from build123d import *

# Parameters (mm, degrees)
F1_DEPTH = 7.25
F2_R     = 3
F3_DEPTH = 25


with BuildPart() as f1:
    # F0 (on Right) → F1 (new body, symmetric)
    with BuildSketch(Plane.YZ):
        with BuildLine():
            Line((14.5, 0), (14.1, 0))
            Line((14.1, 0), (14.1, -0.4))
            Line((14.1, -0.4), (14.1, -1.5))
            Line((14.1, -1.5), (0, -1.5))
            Line((0, -1.5), (0, -1.9))
            Line((0, -1.9), (14.5, -1.9))
            Line((14.5, -1.9), (14.5, -0.4))
            Line((14.5, -0.4), (39.5, -0.4))
            ThreePointArc((39.5, -0.4), (56.431793, 16.531793), (39.5, 33.463586))
            ThreePointArc((39.5, 33.463586), (25.182343, 18.203119), (39.5, 2.942652))
            Line((39.5, 2.942652), (39.5, 3.544018))
            ThreePointArc((39.5, 3.544018), (25.778463, 18.272009), (39.5, 33))
            ThreePointArc((39.5, 33), (56, 16.5), (39.5, 0))
            Line((39.5, 0), (14.5, 0))
        make_face()
    extrude(amount=F1_DEPTH, both=True)

    # F2 (on face) → F3 (cut)
    with BuildSketch(Plane.XY.offset(-1.5)):
        with BuildLine():
            ThreePointArc((6.233854, 1.274401), (3.159757, 0.427693), (0, 0))
            Line((0, 0), (7.25, 0))
            Line((7.25, 0), (7.25, 4.562755))
            Line((7.25, 4.562755), (6.233854, 1.274401))
        make_face()
        with BuildLine():
            ThreePointArc((0, 0), (-3.159757, 0.427693), (-6.233854, 1.274401))
            Line((-6.233854, 1.274401), (-7.25, 4.562755))
            Line((-7.25, 4.562755), (-7.25, 0))
            Line((-7.25, 0), (0, 0))
        make_face()
        with Locations((0, 6)):
            Circle(F2_R)
    extrude(amount=-F3_DEPTH, mode=Mode.SUBTRACT)


solid = f1.part
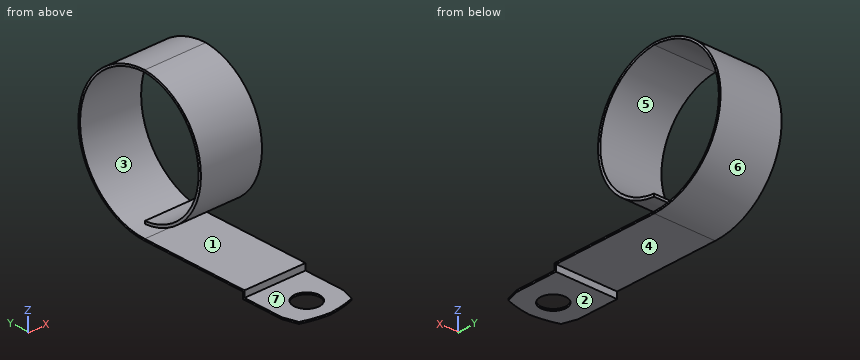
Check sheet for the modelled part. Datum: model origin and axes. Units: mm. Face numbers are marked on the shaded views. A direction names the side the tool comes from. Give positions to 0.01 mm unless a question says otherwise; leave off trailing zeros. Write each loop counter-clockwise with the first axis right and the second up, starting at its lowest first coordinate (ties: lowest second). Pieces come first, ordered by that corner, then holes. Notation, with made-up numbers: (49, 51.5) -> (106, 51.5) arc R18 ccw to (106, 62.5) -> close; hole circle Ø7 at (53.25, 38.5). An arc over 180 degrees is marked (long way). Use one line per item in the form item = value. Start each with the question number.
1. Mould release check, pull along Y, two halves, no side actions. Record for the marked faces 5, 6 and 7: pulls with the +Y half, pulls with the -Y half, needs draft (parallel to the pull), parting line crosses it, or undercut.
2. Access from +Z, -Z, +X, -X, +Y, -Y to the whole of each face (thin tool, end or side, straight path). Record for the marked faces 1, 2, 3 and 4.
3. Thickness scan on line 1 along Z through (x, y) = (-5.25, 48); line 2 along Z through (x, y) = (2.5, 30); line 3 along Z through (x, y) = (-3.75, 43). Record the ranges inside material, lowest first. Write a range as from..to.
4. Section check B-B (z = 5). Record the cut outline in (x, y).
5. Section check D-D (y = 29). Record the cut outline in (x, z), and give its area (3 significant figures).
6. Section check C-C (x = 1.25). Record the cut outline in (y, z), and give its area (3 significant figures).
7. Section check A-A (y = 6). Record the cut outline in (x, z), and give its area (3 significant figures).
8. Go/stop test with flat-tipped pins: P1, Ø8, axis at x = 0, z = 17.5, coming from the -Y side; P2, Ø6, axis at x = -2, y = 6.5, coming from the +Z side; P3, Ø8, axis at x = -2, y = 33, coming from the +Z side; P4, Ø4, axis at y = 39.5, z = 6, coming from the -X side. Record where each tip stops, or that it passes through.
Conclusion:
q1.face_5 = undercut
q1.face_6 = pulls with the +Y half
q1.face_7 = needs draft
q2.face_1 = +X, -X, -Y
q2.face_2 = -Z, +X, -X, +Y, -Y
q2.face_3 = +X, -X
q2.face_4 = -Z, +X, -X, +Y
q3.line_1 = 1.89..2.36, 30.64..31.18
q3.line_2 = -0.4..0, 7.06..7.94, 28.61..29.34
q3.line_3 = -0.03..0.38, 32.62..33.1
q4.outline = (-7.25, 32.76) -> (7.25, 32.76) -> (7.25, 34.07) -> (-7.25, 34.07) -> close; (-7.25, 51.33) -> (7.25, 51.33) -> (7.25, 51.9) -> (-7.25, 51.9) -> close
q5.outline = (-7.25, -0.4) -> (7.25, -0.4) -> (7.25, 0) -> (-7.25, 0) -> close; (-7.25, 8.09) -> (7.25, 8.09) -> (7.25, 9.07) -> (-7.25, 9.07) -> close; (-7.25, 27.48) -> (7.25, 27.48) -> (7.25, 28.31) -> (-7.25, 28.31) -> close
q5.area = 32.0 mm²
q6.outline = (0.12, -1.9) -> (3.27, -1.9) -> (3.27, -1.5) -> (0.12, -1.5) -> close; (8.73, -1.9) -> (14.5, -1.9) -> (14.5, -0.4) -> (39.5, -0.4) arc R16.93 ccw to (39.5, 33.46) arc R15.29 ccw to (39.5, 2.94) -> (39.5, 3.54) arc R14.76 cw to (39.5, 33) arc R16.5 cw to (39.5, 0) -> (14.1, 0) -> (14.1, -1.5) -> (8.73, -1.5) -> close
q6.area = 62.7 mm²
q7.outline = (-7.25, -1.9) -> (-3, -1.9) -> (-3, -1.5) -> (-7.25, -1.5) -> close; (3, -1.9) -> (7.25, -1.9) -> (7.25, -1.5) -> (3, -1.5) -> close
q7.area = 3.40 mm²
q8.P1 = 25.18
q8.P2 = -1.5
q8.P3 = 33.09
q8.P4 = through
